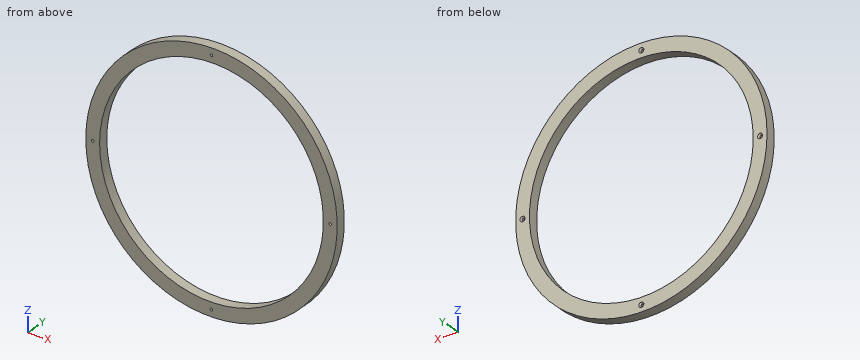
Autodesk Inventor part; units mm, degrees
ref_plane "YZ Plane" through (0, 0, 0) normal (1, 0, 0) x (0, 1, 0)
ref_plane "XZ Plane" through (0, 0, 0) normal (0, 1, 0) x (-1, 0, 0)
ref_plane "XY Plane" through (0, 0, 0) normal (0, 0, 1) x (1, 0, 0)
sketch "Sketch1" plane through (0, 0, 0) normal (0, 1, 0) x (-1, 0, 0)
  circle A0 centre (0, 0) radius 125
  circle A1 centre (0, 0) radius 111.25
  dimension "d0" = 250
  dimension "d1" = 222.5
extrude "Extrusion1" add sketch "Sketch1" along normal blind 10
sketch "Sketch2" plane through (0, 10, 0) normal (0, 1, 0) x (1, 0, 0)
  circle A0 centre (0, 0) radius 118.125
  point P0 (0, 118.125)
  dimension "d4" = 236.25
hole "Hole1" at (0, 10, -118.125) direction (0, -1, 0) diameter 2.5 end through all countersink diameter 5 countersink angle 90
pattern_circular "Circular Pattern1" count 4 over 360 about axis through (0, -10, 0) along (0, 1, 0) of "Hole1"
sketch "Sketch3" plane through (0, 10, 0) normal (0, 1, 0) x (1, 0, 0)
  point P0 (0, 0)
properties part number "OuterBearingTable"
Check sheet for the modelled part. Datum: model origin and axes. Units: mm. Give positions to 0.01 mm unless a question says otherwise; leave off trailing zeros. Write each loop counter-clockwise with the first axis right and the second up, starting at its lowest first coordinate (ties: lowest second). Pieces come first, ordered by that corner, then holes. Notation, with made-up numbers: (51, -9.75) -> (76, -9.75) arc R9 cw to (76, -5.75) -> close; hole circle Ø2 at (73, -28.5). An arc over 180 degrees is marked (long way). Use CSV: the item, a comma, the result in double quotes. Start each with the question number.
Q1. Scan lines: line 1 along Z through (x, y) = (-78, 3.5); line 2 along X through (y, z) = (2.5, -50). Record each from-to range of solid material in increasing order.
Q2. Depth check by flat-ended pin: P1, Ø3, axis at x = 0, z = 118.125, coming from the +Y side; P2, Ø3, axis at x = 14, y = 2.5, coming from the -Z side; P3, Ø1.5, axis at x = -16.5, y = 7, coming from the +Z side; P4, Ø4, axis at x = 118.125, z = 0, coming from the -Y side. Enter the tip coordinate at first touch or a pass-through.
Q3. Cross-section at C-C on x = 22. Enter the section's corners in (y, z).
Q4. Cross-section at B-B on y = 1.5. Enter the section's corners in (x, z) (3 decimals), and give its area (3 significant figures).
Q5. Cross-section at A-A on z = -59.5. Enter the section's corners in (x, y).
Working result:
1,line 1,"z = -97.68 to -79.33, 79.33 to 97.68"
1,line 2,"x = -114.56 to -99.38, 99.38 to 114.56"
2,P1,"stops at y = 9"
2,P2,"stops at z = -124.37"
2,P3,"stops at z = 124"
2,P4,"stops at y = 0"
3,outline,"(0, -123.05) -> (10, -123.05) -> (10, -109.05) -> (0, -109.05) -> close; (0, 109.05) -> (10, 109.05) -> (10, 123.05) -> (0, 123.05) -> close"
4,outline,"circle Ø250 at (0, 0); hole circle Ø2.5 at (-118.125, 0); hole circle Ø222.5 at (0, 0); hole circle Ø2.5 at (0, -118.125); hole circle Ø2.5 at (0, 118.125); hole circle Ø2.5 at (118.125, 0)"
4,area,"10,200 mm^2"
5,outline,"(-109.93, 0) -> (-94, 0) -> (-94, 10) -> (-109.93, 10) -> close; (94, 0) -> (109.93, 0) -> (109.93, 10) -> (94, 10) -> close"
